from build123d import *

# Parameters (mm, degrees)
SKETCH1_W                                           = 70
SKETCH1_H                                           = 70
BOSS_EXTRUDE1_DEPTH                                 = 5
FILLET1_R                                           = 15
CBORE_FOR_M3_HEX_SOCKET_HEAD_CAP_SCREW1_D           = 3.4
CBORE_FOR_M3_HEX_SOCKET_HEAD_CAP_SCREW1_CBORE_D     = 6.5
CBORE_FOR_M3_HEX_SOCKET_HEAD_CAP_SCREW1_CBORE_DEPTH = 3.4
SKETCH5_R                                           = 7.5
CUT_EXTRUDE1_DEPTH                                  = 6
M3_CLEARANCE_HOLE1_D                                = 3.4


with BuildPart() as part:
    # Sketch1 → Boss-Extrude1 (new body)
    with BuildSketch(Plane.XY):
        Rectangle(SKETCH1_W, SKETCH1_H)
    extrude(amount=BOSS_EXTRUDE1_DEPTH)

    # Fillet1
    fillet1_edges = [part.edges().sort_by_distance(p)[0] for p in [
        (35, -35, 2.5),
        (-35, -35, 2.5),
        (-35, 35, 2.5),
        (35, 35, 2.5),
    ]]
    fillet(fillet1_edges, radius=FILLET1_R)

    # CBORE for M3 Hex Socket Head Cap Screw1 (through all)
    with Locations(Plane.XY.offset(5)):
        with Locations((-10.606601718, -10.606601718), (-10.606601718, 10.606601718), (10.606601718, 10.606601718), (10.606601718, -10.606601718)):
            CounterBoreHole(CBORE_FOR_M3_HEX_SOCKET_HEAD_CAP_SCREW1_D / 2, CBORE_FOR_M3_HEX_SOCKET_HEAD_CAP_SCREW1_CBORE_D / 2, CBORE_FOR_M3_HEX_SOCKET_HEAD_CAP_SCREW1_CBORE_DEPTH)

    # Sketch5 → Cut-Extrude1 (cut, through all)
    with BuildSketch(Plane.XY.offset(5)):
        Circle(SKETCH5_R)
    extrude(amount=-CUT_EXTRUDE1_DEPTH, mode=Mode.SUBTRACT)

    # M3 Clearance Hole1 (through all)
    with Locations(Plane.XY.offset(5)):
        with Locations((26, 26), (-26, 26), (-26, -26), (26, -26)):
            Hole(M3_CLEARANCE_HOLE1_D / 2)


solid = part.part
Verification items for the finished model (mm, model axes). A direction names the side the tool comes from. Give positions to 0.01 mm unless a question says otherwise; leave off trailing zeros. Write each loop counter-clockwise with the first axis right and the second up, starting at its lowest first coordinate (ties: lowest second). Pieces come first, ordered by that corner, then holes. Notation, with made-up numbers: (1, 53.25) - (58, 53.25) arc R26 ccw to (58, 70.25) - close; hole circle Ø3 at (84, -9.5). An arc over 180 degrees is marked (long way). Answer as CSV lines item,"result". Start each with the question number.
1. Depth check by flat-ended pin: pin 1 (2.5 mm diameter, centred on x = -26, y = 26, fed in from -Z); pin 2 (3 mm diameter, centred on x = 9, y = -10, fed in from +Z). Enter the tip coordinate at first touch or a pass-through.
2. Sectioned sample at D-D (y = 26). Record the boundary of the cut face in (x, z).
3. Sectioned sample at A-A (x = 0). Record the boundary of the cut face in (y, z).
4. Thickness scan on line 1 (Y direction, x = 26, z = 3.95); line 2 (Y direction, x = -10, z = 3.9); line 3 (X direction, y = -13.5, z = 3.5). Record the ranges inside material, lowest first.
5. Set-up check for faces 4 (the face through (30.49, -30.72, 2.54)), 5 (the face through (-9, 9, 1.6)): record each of +Z, -Z, +X, -X, +Y, -Y from which the full face is reachable in a straight line by a thin tool's end or side.
6. Sectioned sample at C-C (z = 3.7). Count the separate pieces of the cut face and the enclosed holes in it, then the cut area to 3 significant figures.
7. Draft check along X on faces 1 (the face through (0, -35, 2)), 2 (the face through (-11.31, -13.78, 3.32)), 3 (the face through (-30.72, 30.49, 2.54)). Enter one of: pulls with the +X half, pulls with the -X half, needs draft (parallel to the pull), parting line crosses it, or undercut.
Derived:
1,pin 1,"through"
1,pin 2,"z = 1.6"
2,outline,"(-33.75, 0) - (-27.7, 0) - (-27.7, 5) - (-33.75, 5) - close; (-24.3, 0) - (24.3, 0) - (24.3, 5) - (-24.3, 5) - close; (27.7, 0) - (33.75, 0) - (33.75, 5) - (27.7, 5) - close"
3,outline,"(-35, 0) - (-7.5, 0) - (-7.5, 5) - (-35, 5) - close; (7.5, 0) - (35, 0) - (35, 5) - (7.5, 5) - close"
4,line 1,"-33.75 to -27.7, -24.3 to 24.3, 27.7 to 33.75"
4,line 2,"-35 to -13.8, -7.41 to 7.41, 13.8 to 35"
4,line 3,"-35 to -12.09, -9.13 to 9.13, 12.09 to 35"
5,face 4,"+Z, -Z, +X, -Y"
5,face 5,"+Z"
6,separate pieces,"1"
6,enclosed holes,"9"
6,area,"4,360 mm²"
7,face 1,"needs draft"
7,face 2,"undercut"
7,face 3,"pulls with the -X half"
